For this review, take the finished solid that the model builds, in its own axes (mm). Face numbers are marked on the shaded views. A direction names the side the tool comes from. Give positions to 0.01 mm unless a question says otherwise; leave off trailing zeros. Order: outer loops, then holes, each group sorted by start corner. A loop starts at its lowest first (then second) coordinate and runs counter-clockwise, first axis right, second up.
Item 1: Machinability: for the marked faces 4, 5, 6, 7 and 8, which of the approach directions +Z, -Z, +X, -X, +Y, -Y give a long, thin tool a straight path to every point of the face, cutting with its end or side? Answer none if there is none.
Item 2: Consider section D-D (z = -33). Give the boundary of the cut face in (x, y), plus the area to 3 significant figures.
Item 3: The part is to be moulded in two halves that separate along X. For the marked faces 1, 2 and 3, say which applies: released by +X, released by -X, zero draft, split by the parting line, or undercut.
Item 4: For probe 1 along X at (y, z) = (154.5, -150); probe 2 along Z at (x, y) = (-120, 8); probe 3 along Z at (x, y) = (-120, 155.25), list the stretches that pass through material, from the lowest coordinate up.
Item 5: For P1, Ø22.5, axis at x = -120, z = -30, coming from the +Y side; P2, Ø2.5, axis at y = 45, z = -103, coming from the -X side; P3, Ø6, axis at x = -92, y = 85, coming from the -Z side; P4, Ø12, axis at x = -88.5, z = -136.5, coming from the +Y side, all flat-tipped, find the tip position at first contact; note any pin that passes through.
Item 6: Consider section C-C (y = 150). Give the boundary of the cut face in (x, z).
Item 7: Consider section B-B (x = -120). Give the boundary of the cut face in (y, z).
Item 8: Consider section A-A (z = -270). Give the boundary of the cut face in (x, y), plus the area to 3 significant figures.
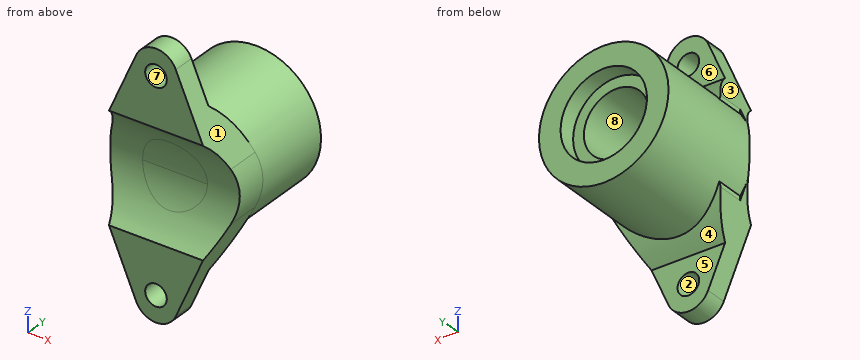
Autodesk Inventor part; units mm, degrees
ref_plane "XZ Plane" through (0, 0, 0) normal (0, 1, 0) x (-1, 0, 0)
ref_plane "XY Plane" through (0, 0, 0) normal (0, 0, 1) x (1, 0, 0)
sketch "Sketch1" plane through (0, 0, 0) normal (1, 0, 0) x (0, 1, 0)
  point P0 (0, 0)
sketch "Sketch2" plane through (0, 0, 0) normal (1, 0, 0) x (0, 1, 0)
  line L0 (0, 0) -> (160, 0)
  line L1 (160, 0) -> (160, -300)
  line L2 (160, -300) -> (0, -300)
  line L3 (0, -300) -> (0, 0)
  dimension "d0" = 300
  dimension "d1" = 160
extrude "Extrusion1" add sketch "Sketch2" against normal blind 240
sketch "Sketch3" plane through (0, 160, 0) normal (0, 1, 0) x (1, 0, 0)
  line L0 (-240, 300) -> (-240, 0)
  line L1 (-240, 150) -> (0, 150)
  line L2 (0, 0) -> (0, 300)
  line L3 (0, 0) -> (-240, 0)
  line L4 (-120, 0) -> (-120, 300) construction
  circle A0 centre (-120, 150) radius 75
  circle A1 centre (-120, 150) radius 50
  circle A2 centre (-120, 150) radius 37.5
  line L5 (-120, 30) -> (-120, 270) construction
  circle A3 centre (-120, 270) radius 12.5
  circle A4 centre (-120, 30) radius 12.5
  line L6 (0, 300) -> (-240, 300)
  line L7 (-188.7386, 180) -> (-142.9129, 285)
  line L8 (-51.2614, 180) -> (-97.0871, 285)
  arc A5 (-97.0871, 285) -> (-142.9129, 285) centre (-120, 275) ccw
  line L9 (-188.7386, 120) -> (-142.9129, 15)
  line L10 (-51.2614, 120) -> (-97.0871, 15)
  arc A6 (-142.9129, 15) -> (-97.0871, 15) centre (-120, 25) ccw
  point P0 (-120, 300)
  point P1 (-120, 300)
  point P2 (-120, 0)
  dimension "d4" = 150
  dimension "d5" = 100
  dimension "d6" = 75
  dimension "d7" = 240
  dimension "d8" = 25
  dimension "d9" = 25
  dimension "d13" = 25
extrude "Extrusion2" cut sketch "Sketch3" against normal blind 160 contours L6 A5 L7 A0 L1 L0 | L1 A0 L9 A6 L3 L0 | L6 L2 L1 A0 L8 A5 | A6 L10 A0 L1 L2 L3
extrude "Extrusion3" cut sketch "Sketch3" against normal blind 160 contours A3 | A4
extrude "Extrusion4" cut sketch "Sketch3" against normal blind 160 contours A2 L1 | L1 A2
extrude "Extrusion5" cut sketch "Sketch3" against normal blind 20 contours A1 L1 A2 | L1 A2 A1
ref_plane "Work Plane1" through (-45, 160, -150) normal (1, 0, 0) x (0, 1, 0)
sketch "Sketch4" plane through (-45, 160, -150) normal (1, 0, 0) x (0, 1, 0)
  circle A0 centre (-209.6065, 0) radius 80
  line L0 (-20, -37.5) -> (-160, -37.5)
  line L1 (-160, -37.5) -> (-160, 37.5)
  line L2 (-20, -37.5) -> (-160, -37.5)
  line L3 (-20, -37.5) -> (-20, 37.5)
  line L4 (-20, 37.5) -> (-160, 37.5)
  line L5 (-160, 135) -> (-160, 30)
  line L6 (0, -30) -> (0, 30)
  line L7 (0, 0) -> (-160, 0)
  line L8 (-160, 150) -> (-160, 70)
  line L9 (-160, 150) -> (-160, 90)
  line L10 (-160, 150) -> (-135, 150)
  line L11 (-160, 150) -> (0, 150)
  line L12 (-135, 150) -> (-135, -149.8181) construction
  line L13 (-160, 90) -> (-135, 90) construction
  circle A1 centre (-209.6065, 0) radius 116.9023
  line L14 (-160, 105.8552) -> (-160, 62.763) construction
  line L15 (-160, -62.763) -> (-160, -105.8552) construction
  line L16 (-160, 0) -> (-160, -105.8552)
  line L17 (-160, -132.5) -> (-160, -107.5)
  point P0 (-160, -62.763)
  point P1 (-160, 105.8552)
  dimension "d22" = 160
  dimension "d23" = 80
  dimension "d24" = 0
  dimension "d25" = 70
  dimension "d26" = 60
  dimension "d31" = 25
extrude "Extrusion6" cut sketch "Sketch4" against normal blind 150 contours L7 L1 L4 A0 | A0 L0 L1 L7 | L4 L5 A0 | A0 L16 L0 | L1 L16 A0 L5
extrude "Extrusion7" cut sketch "Sketch3" against normal blind 135 contours A5 L8 A0 L7 | A6 L9 A0 L10
extrude "Extrusion8" add sketch "Sketch4" against normal blind 135 contours L7 A1 L0 A0 | A0 L4 A1 L7 | A0 L5 A1 L4 | L0 A1 L16 A0 | A0 L16 A1 L5
extrude "Extrusion9" cut sketch "Sketch4" against normal blind 135 contours A0 L16 A1 L5
extrude "Extrusion10" cut sketch "Sketch3" against normal blind 200 contours L6 A5 L7 A0 L1 L0 | L1 A0 L9 A6 L3 L0 | L6 L2 L1 A0 L8 A5 | A6 L10 A0 L1 L2 L3
properties part number "Baitap4"
Resolved:
1. face 4: -Z, +Y
1. face 5: -Z, +X, -X, +Y
1. face 6: +Z, +X, -X, +Y
1. face 7: +Y, -Y
1. face 8: +Y
2. outline: (-150.77, 0) - (-132.13, 0) - (-132.13, 25) - (-150.77, 25) - close; (-107.87, 0) - (-89.23, 0) - (-89.23, 25) - (-107.87, 25) - close
2. area: 932 mm2
3. face 1: released by +X
3. face 2: undercut
3. face 3: released by -X
4. probe 1: x = -195 to -170, -70 to -45
4. probe 2: z = -300 to -282.5, -257.5 to -205.51, -94.49 to -42.5, -17.5 to 0
4. probe 3: z = -225 to -200, -100 to -75
5. P1: passes through
5. P2: stops at x = -180
5. P3: stops at z = -220.71
5. P4: stops at y = 140
6. outline: circle Ø150 at (-120, -150); hole circle Ø100 at (-120, -150)
7. outline: (0, -300) - (25, -300) - (25, -282.5) - (0, -282.5) - close; (0, -257.5) - (25, -257.5) - (25, -240) arc R116.9 ccw to (40.07, -225) - (160, -225) - (160, -200) - (140, -200) - (140, -187.5) - (61.12, -187.5) arc R116.9 ccw to (61.12, -112.5) - (140, -112.5) - (140, -100) - (160, -100) - (160, -75) - (40.07, -75) arc R116.9 ccw to (25, -60) - (25, -42.5) - (0, -42.5) - (0, -87.24) arc R80 cw to (0, -212.76) - close; (0, -17.5) - (25, -17.5) - (25, 0) - (0, 0) - close
8. outline: (-149.46, 0) - (-132.5, 0) - (-132.5, 25) - (-149.46, 25) - close; (-107.5, 0) - (-90.54, 0) - (-90.54, 25) - (-107.5, 25) - close
8. area: 848 mm2
